Here's how the part is built. I have some questions about the finished solid (model axes, mm). Face numbers are marked on the shaded views. A direction names the side the tool comes from. Give positions to 0.01 mm unless a question says otherwise; leave off trailing zeros. Write each loop counter-clockwise with the first axis right and the second up, starting at its lowest first coordinate (ties: lowest second). Pieces come first, ordered by that corner, then holes. Notation, with made-up numbers: M -37.5,-7.75 L -21.5,-7.75 A36 cw -21.5,31.25 Z; hole C -5.5,46 d3. An arc over 180 degrees is marked long. Answer as CSV lines item,"result". Start each with the question number.
Q1. Thinking about a two-plate mould opening in Y: for the marked faces 1, 2, 3 and 4, which applies, +Y half, -Y half, draft (parallel to the pull), parting line (faces both ways), or undercut?
Q2. For pin 1 (1.1 mm diameter, centred on y = 8.5, z = 4.5, fed in from +X); pin 2 (0.8 mm diameter, centred on y = -9, z = 3, fed in from -X); pin 3 (1.4 mm diameter, centred on y = -9, z = 3.5, fed in from +X), each with a flat end and sliding along its axis, tell me the tip position at first contact or that it passes through.
Q3. On a 3-axis mill with a long thin cutter (end or side, diameter ignored), from which of +Z, -Z, +X, -X, +Y, -Y can I reach the whole of each face in a straight line? I mean the marked faces 5 and 6. Say none if no direction works.
Q4. Suppose I cut it at D-D (y = 9.5). Write out the boundary of the cut face in (x, z), then the cut area to 3 significant figures.
Q5. If I drill on line 1 along X through (y, z) = (-7.5, 2.75) (3 decimals); line 2 along Y through (x, z) = (1.75, 0.5); line 3 along X through (y, z) = (-1, 5), over which ranges is the centre line in solid material (lowest first)?
Q6. Suppose I cut it at B-B (x = 0). Write out the boundary of the cut face in (y, z).
Q7. Suppose I cut it at C-C (y = 2). Write out the boundary of the cut face in (x, z).
Q8. Suppose I cut it at A-A (z = 1.5). Write out the boundary of the cut face in (x, y) (3 decimals).
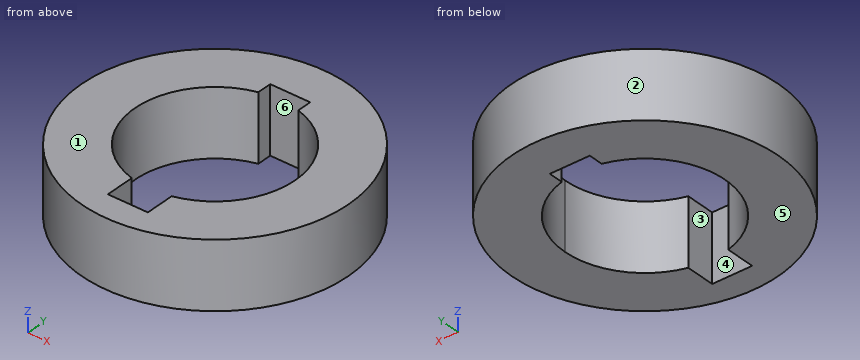
```python
from build123d import *

# Parameters (mm, degrees)
F0_R     = 12.7
F1_DEPTH = 6.35
F2_W     = 3.81
F2_H     = 1.39192
F3_DEPTH = 6.35


with BuildPart() as f1:
    # F0 (on Top) → F1 (new body)
    with BuildSketch(Plane.XY):
        Circle(F0_R)
        with BuildLine():
            ThreePointArc((1.905, 7.378033), (6.024139, 4.666278), (7.62, 0))
            ThreePointArc((7.62, 0), (6.024139, -4.666278), (1.905, -7.378033))
            Line((1.905, -7.378033), (1.905, -10.16))
            Line((1.905, -10.16), (-1.905, -10.16))
            Line((-1.905, -10.16), (-1.905, -7.378033))
            ThreePointArc((-1.905, -7.378033), (-7.62, 0), (-1.905, 7.378033))
            Line((-1.905, 7.378033), (-1.905, 10.16))
            Line((-1.905, 10.16), (1.905, 10.16))
            Line((1.905, 10.16), (1.905, 7.378033))
        make_face(mode=Mode.SUBTRACT)
    extrude(amount=F1_DEPTH)

    # F2 (on face) → F3 (join)
    with BuildSketch(Plane.XY.offset(6.35)):
        with Locations((0, 9.46404)):
            Rectangle(F2_W, F2_H)
    extrude(amount=-F3_DEPTH)


solid = f1.part
```
Resolved:
1,face 1,"draft"
1,face 2,"parting line"
1,face 3,"undercut"
1,face 4,"undercut"
2,pin 1,"x = 9.9"
2,pin 2,"x = -9.35"
2,pin 3,"x = 9.61"
3,face 5,"-Z, +X, -X, +Y, -Y"
3,face 6,"+Z, -Z"
4,outline,"M -8.43,0 L 8.43,0 L 8.43,6.35 L -8.43,6.35 Z"
4,area,"107 mm^2"
5,line 1,"-10.249 to -1.905, 1.905 to 10.249"
5,line 2,"-12.58 to -10.16, 8.77 to 12.58"
5,line 3,"-12.66 to -7.55, 7.55 to 12.66"
6,outline,"M -12.7,0 L -10.16,0 L -10.16,6.35 L -12.7,6.35 Z; M 8.77,0 L 12.7,0 L 12.7,6.35 L 8.77,6.35 Z"
7,outline,"M -12.54,0 L -7.35,0 L -7.35,6.35 L -12.54,6.35 Z; M 7.35,0 L 12.54,0 L 12.54,6.35 L 7.35,6.35 Z"
8,outline,"C 0,0 d25.4; hole M -1.905,-10.16 L 1.905,-10.16 L 1.905,-7.378 A7.62 ccw 1.905,7.378 L 1.905,8.768 L -1.905,8.768 L -1.905,7.378 A7.62 ccw -1.905,-7.378 Z"
